Geometry check sheet. Reference: the model listing, model coordinates, mm. A direction names the side the tool comes from. Round coordinates to 2 decimals unless told otherwise and drop trailing zeros. Write each loop counter-clockwise with the first axis right and the second up, starting at its lowest first coordinate (ties: lowest second). Pieces come first, ordered by that corner, then holes. Notation, with made-up numbers: M 8.25,49 L 27.25,49 A20 ccw 27.25,58 Z; hole C 40.25,5.5 d8. An arc over 180 degrees is marked long. Use a Markdown table: item, result.
```python
from build123d import *

# Parameters (mm, degrees)
SKETCH1_R               = 15
BASE_EXTRUDE_DEPTH      = 5
CHAMFER1_2_OUTLINE_W    = 10
CHAMFER1_2_OUTLINE_H    = 80
CHAMFER2_SIZE           = 4
CUT_EXTRUDE1_DEPTH      = 74.813887582
CUT_EXTRUDE1_DEPTH_BACK = 74.813887582
SKETCH3_R               = 2.5


with BuildPart() as part:
    # Sketch1 → Base-Extrude (new body)
    with BuildSketch(Plane.XY):
        Circle(SKETCH1_R)
    extrude(amount=-BASE_EXTRUDE_DEPTH)

    # Chamfer1: read off the stored shape, not the designer's step
    # Chamfer1 outline → Chamfer1 (revolve, cut)
    with BuildSketch(Plane.XZ):
        Polygon((15, -3), (13, -5), (15, -5), align=None)
    revolve(axis=Axis((0, 0, 0), (0, 0, 1)), mode=Mode.SUBTRACT)

    # Chamfer1 2 outline → Chamfer1 2 (revolve)
    with BuildSketch(Plane.XZ):
        with Locations((5, 40)):
            Rectangle(CHAMFER1_2_OUTLINE_W, CHAMFER1_2_OUTLINE_H)
    revolve(axis=Axis((0, 0, 0), (0, 0, 1)))

    # Chamfer2
    chamfer2_edges = [part.edges().sort_by_distance(p)[0] for p in [
        (-10, 0, 80),
    ]]
    chamfer(chamfer2_edges, length=CHAMFER2_SIZE)

    # Sketch3 → Cut-Extrude1 (cut, two sides: drawn at the far end of the back side and taken through both)
    with BuildSketch(Plane(origin=(0, 0, 9.3), x_dir=(0, -1, 0), z_dir=(1, 0, 0)).offset(-CUT_EXTRUDE1_DEPTH_BACK)):
        with Locations(Location((0, -62.7, 0), (0, 0, 270))):
            Circle(SKETCH3_R)
    extrude(amount=CUT_EXTRUDE1_DEPTH + CUT_EXTRUDE1_DEPTH_BACK, mode=Mode.SUBTRACT)


solid = part.part
```
Item 1: Access from +Z, -Z, +X, -X, +Y, -Y to the whole of each face (thin tool, end or side, straight path). Record for faces 4 (the face through (9.237, -3.83, 38.532)), 5 (the face through (0, 0, -5)).
Outcome:
| item | result |
|---|---|
| face 4 | +Z |
| face 5 | -Z, +X, -X, +Y, -Y |
Item 2: Go/stop test with flat-tipped pins: pin 1 (6 mm diameter, centred on y = 0, z = 72, fed in from +X); pin 2 (1.5 mm diameter, centred on x = -9.5, z = 32.5, fed in from +Y); pin 3 (5 mm diameter, centred on y = 11.5, z = 66.5, fed in from -X). Record where each tip stops, or that it passes through.
Outcome:
| item | result |
|---|---|
| pin 1 | stops at x = 10 |
| pin 2 | stops at y = 4.84 |
| pin 3 | stops at x = -4.36 |
Item 3: Material ranges on line 1 along Z through (x, y) = (7.5, 8.25); line 2 along X through (y, z) = (0, 3.5); line 3 along Y through (x, z) = (4.5, 72), recorded low to high. Write a range as from..to.
Outcome:
| item | result |
|---|---|
| line 1 | z = -5..0 |
| line 2 | x = -10..10 |
| line 3 | y = -8.93..-2.5, 2.5..8.93 |
Item 4: Mould release check, pull along Z, two halves, no side actions. Record for faces 1 (the face through (-14.985, 0.66, -1.479)), 2 (the face through (3, -10, 0)), 3 (the face through (-0.1, 1.5, 70)): +Z half, -Z half, draft (parallel to the pull), parting line (faces both ways), or undercut.
Outcome:
| item | result |
|---|---|
| face 1 | draft |
| face 2 | +Z half |
| face 3 | undercut |
Item 5: Cross-section at C-C, the plane z = 31.5. Record the cut outline in (x, y), and give its area (3 significant figures).
Outcome:
| item | result |
|---|---|
| outline | C 0,0 d20 |
| area | 314 mm2 |
Item 6: Cross-section at D-D, the plane z = 72. Record the cut outline in (x, y), and give its area (3 significant figures).
Outcome:
| item | result |
|---|---|
| outline | M -9.68,-2.5 A10 ccw 9.68,-2.5 Z; M -9.68,2.5 L 9.68,2.5 A10 ccw Z |
| area | 215 mm2 |
Item 7: Cross-section at A-A, the plane y = 0. Record the cut outline in (x, z).
Outcome:
| item | result |
|---|---|
| outline | M -15,-3 L -13,-5 L 13,-5 L 15,-3 L 15,0 L 10,0 L 10,69.5 L -10,69.5 L -10,0 L -15,0 Z; M -10,74.5 L 10,74.5 L 10,76 L 6,80 L -6,80 L -10,76 Z |
Item 8: Cross-section at B-B, the plane x = 0. Record the cut outline in (y, z), and give its area (3 significant figures).
Outcome:
| item | result |
|---|---|
| outline | M -15,-3 L -13,-5 L 13,-5 L 15,-3 L 15,0 L 10,0 L 10,76 L 6,80 L -6,80 L -10,76 L -10,0 L -15,0 Z; hole C 0,72 d5 |
| area | 1,710 mm2 |
